Design review of the part built by this model. Coordinates are the model's own, in mm. Coordinates: 2 decimals unless noted, no trailing zeros. Loops run counter-clockwise (first coordinate to the right, second up) from the corner with the lowest first, then second, coordinate; pieces in that order, holes last. Notation, with made-up numbers: (-7, 48.25) - (17, 48.25) arc R25 ccw to (17, 61.25) - close; hole circle Ø1 at (11, 20). An arc over 180 degrees is marked (long way). Answer in a Markdown table with one row per item. Add a question column.
(1) We need section A-A, the plane y = 0.5. Write out the cut boundary in (x, z).
(2) To check wall thickness, follow L1, parallel to Z at x = 10, y = 10.25; L2, parallel to X at y = 4.75, z = 3.5; L3, parallel to X at y = 3, z = 6.5. State the ranges of each line that lie inside material, in increasing order. Write a range as [from, to].
(3) We need section C-C, the plane x = 13.75. Write out the cut boundary in (y, z), plus the area to 3 significant figures.
(4) We need section B-B, the plane z = 11.25. Write out the cut boundary in (x, y), plus the area to 3 significant figures.
(5) Clearance check with flat-ended pins moving along their axes: pin 1 (0.6 mm diameter, centred on y = 2, z = -2.5, fed in from +X); pin 2 (1.5 mm diameter, centred on x = 4, y = 2.5, fed in from -Z); pin 3 (0.6 mm diameter, centred on x = 6.5, z = -1.5, fed in from +Y). State where each tip first meets the part, or that it passes through.
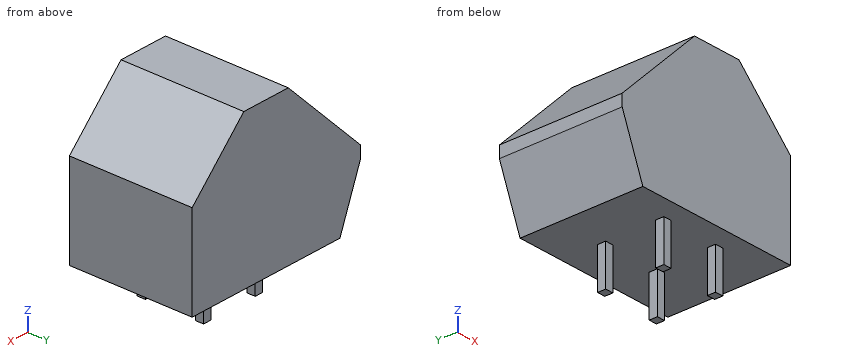
from build123d import *

# Parameters (mm, degrees)
SKETCH_1_W      = 16.3
SKETCH_1_H      = 10.55
EXTRUDE_1_DEPTH = 13
CHAMFER_1_SIZE  = 5
CHAMFER_3_SIZE  = 2
CHAMFER_3_SIZE2 = 5
CHAMFER_4_SIZE  = 7
SKETCH_2_W      = 0.7
SKETCH_2_H      = 0.7
EXTRUDE_2_DEPTH = 3.5


with BuildPart() as part:
    # Эскиз1 → Бобышка-Вытянуть1 (new body)
    with BuildSketch(Plane.XY):
        with Locations((8.15, 5.275)):
            Rectangle(SKETCH_1_W, SKETCH_1_H)
    extrude(amount=EXTRUDE_1_DEPTH)

    # Фаска1
    chamfer_1_edges = [part.edges().sort_by_distance(p)[0] for p in [
        (16.3, 5.275, 13),
    ]]
    chamfer(chamfer_1_edges, length=CHAMFER_1_SIZE)

    # Фаска3
    chamfer_3_edges = [part.edges().sort_by_distance(p)[0] for p in [
        (0, 5.275, 0),
    ]]
    chamfer_3_side = [part.faces().sort_by_distance(p)[0] for p in [
        (8.15, 5.275, 0),
    ]]
    chamfer(chamfer_3_edges, length=CHAMFER_3_SIZE, length2=CHAMFER_3_SIZE2, reference=chamfer_3_side[0])

    # Фаска4
    chamfer_4_edges = [part.edges().sort_by_distance(p)[0] for p in [
        (0, 5.275, 13),
    ]]
    chamfer(chamfer_4_edges, length=CHAMFER_4_SIZE)

    # Эскиз2 → Бобышка-Вытянуть2 (add)
    with BuildSketch(Plane(origin=(0, 0, 0), x_dir=(-1, 0, 0), z_dir=(0, 0, -1))):
        with Locations((-6.3, 2.05)):
            Rectangle(SKETCH_2_W, SKETCH_2_H)
        with Locations((-6.3, 7.05)):
            Rectangle(SKETCH_2_W, SKETCH_2_H)
        with Locations((-11.3, 2.05)):
            Rectangle(SKETCH_2_W, SKETCH_2_H)
        with Locations((-11.3, 7.05)):
            Rectangle(SKETCH_2_W, SKETCH_2_H)
    extrude(amount=EXTRUDE_2_DEPTH)


solid = part.part
Responses:
| question | item | result |
|---|---|---|
| 1 | outline | (0, 5) - (2, 0) - (16.3, 0) - (16.3, 8) - (11.3, 13) - (7, 13) - (0, 6) - close |
| 2 | L1 | z = [0, 13] |
| 2 | L2 | x = [0.6, 16.3] |
| 2 | L3 | x = [0.5, 16.3] |
| 3 | outline | (0, 0) - (10.55, 0) - (10.55, 10.55) - (0, 10.55) - close |
| 3 | area | 111 mm2 |
| 4 | outline | (5.25, 0) - (13.05, 0) - (13.05, 10.55) - (5.25, 10.55) - close |
| 4 | area | 82.3 mm2 |
| 5 | pin 1 | stops at x = 11.65 |
| 5 | pin 2 | stops at z = 0 |
| 5 | pin 3 | stops at y = 7.4 |
